```python
from build123d import *

# Parameters (mm, degrees)
SKETCH_1_R          = 2.9
EXTRUDE_1_DEPTH     = 40
SKETCH_2_R          = 10
EXTRUDE_2_DEPTH     = 2
SKETCH_3_R          = 1.75
CUT_EXTRUDE_1_DEPTH = 3


with BuildPart() as part:
    # 草图1 → 凸台-拉伸1 (new body)
    with BuildSketch(Plane(origin=(0, 0, 0), x_dir=(1, 0, 0), z_dir=(0, 1, 0))):
        with Locations(Location((0, 0, 0), (0, 0, 270))):
            Circle(SKETCH_1_R)
    extrude(amount=EXTRUDE_1_DEPTH)

    # 草图2 → 凸台-拉伸2 (add)
    with BuildSketch(Plane.XZ):
        with Locations(Location((0, 0, 0), (0, 0, 270))):
            Circle(SKETCH_2_R)
    extrude(amount=-EXTRUDE_2_DEPTH)

    # 草图3 → 切除-拉伸1 (cut)
    with BuildSketch(Plane(origin=(0, 2, 0), x_dir=(1, 0, 0), z_dir=(0, 1, 0))):
        with Locations(Location((-3.814504668, -5.869398434, 0), (0, 0, 270))):
            Circle(SKETCH_3_R)
        with Locations(Location((-5.869398434, 3.814504668, 0), (0, 0, 270))):
            Circle(SKETCH_3_R)
        with Locations(Location((3.814504668, 5.869398434, 0), (0, 0, 270))):
            Circle(SKETCH_3_R)
        with Locations(Location((5.869398434, -3.814504668, 0), (0, 0, 270))):
            Circle(SKETCH_3_R)
    extrude(amount=-CUT_EXTRUDE_1_DEPTH, mode=Mode.SUBTRACT)


solid = part.part
```
CAD build for the part. Positions are in the model's coordinates, mm. A direction names the side the tool comes from. Give positions to 0.01 mm unless a question says otherwise; leave off trailing zeros. Order: outer loops, then holes, each group sorted by start corner. A loop starts at its lowest first (then second) coordinate and runs counter-clockwise, first axis right, second up.
(1) Saw through at C-C, the plane x = 4.75. Give the cut face in (y, z).
(2) Saw through at D-D, the plane z = 0. Give the cut face in (x, y).
(3) Saw through at B-B, the plane x = 0. Give the cut face in (y, z).
(4) Tool access for faces 4 (the cylindrical face through (2.262, 1.014, -5.062)), 5 (the cylindrical face through (0.1, 20.7, -2.9)): list every direction of +Z, -Z, +X, -X, +Y, -Y with a clear straight run to the whole face (end or side of a thin tool).
(5) Drill centre lines: L1, parallel to Y at x = -2.75, z = -3.25; L2, parallel to X at y = 19, z = 0; L3, parallel to X at y = 28, z = 1. Where is each one in solid material? Low to high.
(6) Saw through at A-A, the plane z = -6.75. Give the cut face in (x, y).
(7) Flat gauge pins, fed straight in: pin 1 (1.5 mm diameter, centred on x = -2, y = 23.5, fed in from -Z); pin 2 (3 mm diameter, centred on x = -5.87, z = -3.81, fed in from +Y); pin 3 (8 mm diameter, centred on x = 3.5, y = 30, fed in from -Z); pin 4 (6 mm diameter, centred on y = 35, z = 4, fed in from +X). Where does each tip first touch, or does it go through?
(8) Mould opens along Z. For faces 1 (the cylindrical face through (-6.934, 1.014, -5.203)), 2 (the flat face through (-2.1, 2, 2.4)), 3 (the cylindrical face through (-9.76, 0.99, 2.17)) say: released by +Z, released by -Z, zero draft, split by the parting line, or undercut.
Results found:
1. outline: (0, -8.8) - (2, -8.8) - (2, -7.35) - (0, -7.35) - close; (0, -4.39) - (2, -4.39) - (2, 2.47) - (0, 2.47) - close; (0, 5.16) - (2, 5.16) - (2, 8.8) - (0, 8.8) - close
2. outline: (-10, 0) - (10, 0) - (10, 2) - (2.9, 2) - (2.9, 40) - (-2.9, 40) - (-2.9, 2) - (-10, 2) - close
3. outline: (0, -10) - (2, -10) - (2, -2.9) - (40, -2.9) - (40, 2.9) - (2, 2.9) - (2, 10) - (0, 10) - close
4. face 4: +Y, -Y
4. face 5: +Y
5. L1: y = 0 to 2
5. L2: x = -2.9 to 2.9
5. L3: x = -2.72 to 2.72
6. outline: (-7.38, 0) - (2.3, 0) - (2.3, 2) - (-7.38, 2) - close; (5.33, 0) - (7.38, 0) - (7.38, 2) - (5.33, 2) - close
7. pin 1: stops at z = -2.62
7. pin 2: passes through
7. pin 3: stops at z = -2.9
7. pin 4: stops at x = 2.72
8. face 1: undercut
8. face 2: zero draft
8. face 3: split by the parting line
